Study the drawing (mm; zero at the part's minimum x, y, z) and answer. Round coordinates to 2 decimals unless told otherwise and drop trailing zeros. Write each loop counter-clockwise with the first axis right and the second up, starting at its lowest first coordinate (ties: lowest second). Pieces come first, ordered by that corner, then holes.
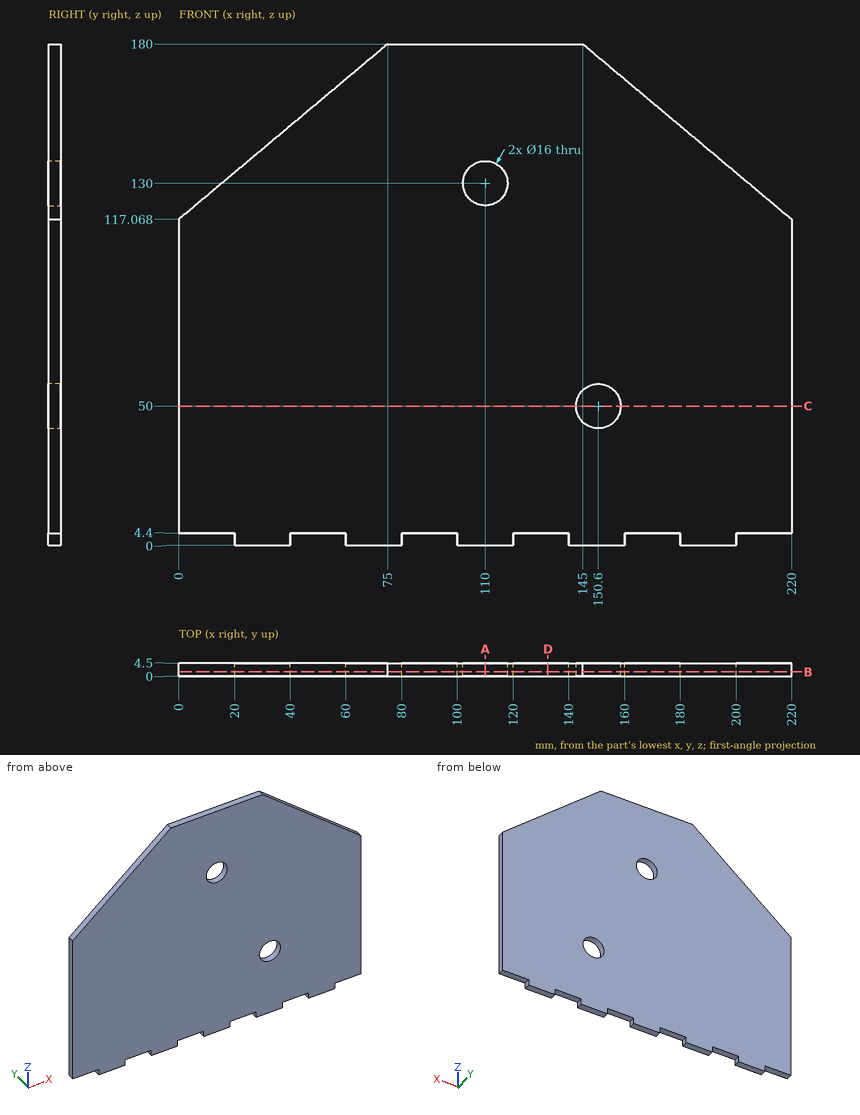
1. Section D-D on x = 132.5 is taken. Determine the outline of the cut face in (y, z).
Geometry says:
outline: (0, 4.4) - (4.5, 4.4) - (4.5, 180) - (0, 180) - close
2. Given pin 1 (1.3 mm diameter, centred on y = 2.5, z = 2.5, fed in from -X); pin 2 (2 mm diameter, centred on x = 172.5, y = 1, fed in from -Z); pin 3 (1.5 mm diameter, centred on y = 4, z = 155.5, fed in from +X), each flat-ended and moving along its own axis, determine where each tip first touches the part or whether it passes through.
Geometry says:
pin 1: stops at x = 20
pin 2: stops at z = 4.4
pin 3: stops at x = 175.09
3. Section B-B on y = 1.5 is taken. Determine the outline of the cut face in (x, z), plus the area to 4 significant figures.
Geometry says:
outline: (0, 4.4) - (20, 4.4) - (20, 0) - (40, 0) - (40, 4.4) - (60, 4.4) - (60, 0) - (80, 0) - (80, 4.4) - (100, 4.4) - (100, 0) - (120, 0) - (120, 4.4) - (140, 4.4) - (140, 0) - (160, 0) - (160, 4.4) - (180, 4.4) - (180, 0) - (200, 0) - (200, 4.4) - (220, 4.4) - (220, 117.07) - (145, 180) - (75, 180) - (0, 117.07) - close; hole circle Ø16 at (110, 130); hole circle Ø16 at (150.6, 50)
area: 33,950 mm2
4. Section A-A on x = 110 is taken. Determine the outline of the cut face in (y, z).
Geometry says:
outline: (0, 0) - (4.5, 0) - (4.5, 122) - (0, 122) - close; (0, 138) - (4.5, 138) - (4.5, 180) - (0, 180) - close
5. Straight lines are drawn through the part: line 1 along X through (y, z) = (3.3, 50); line 2 along Z through (x, y) = (25, 3.7) (1 decimal); line 3 along Z through (x, y) = (138, 4.35). For each, find the intervals that lie inside material, in ascending order.
Geometry says:
line 1: x = 0 to 142.6, 158.6 to 220
line 2: z = 0 to 138
line 3: z = 4.4 to 180
6. Section C-C on z = 50 is taken. Determine the outline of the cut face in (x, y).
Geometry says:
outline: (0, 0) - (142.6, 0) - (142.6, 4.5) - (0, 4.5) - close; (158.6, 0) - (220, 0) - (220, 4.5) - (158.6, 4.5) - close
